Part model, mm, in its own coordinate system. Face numbers are marked on the shaded views. A direction names the side the tool comes from. Coordinates: 2 decimals unless noted, no trailing zeros. Loops run counter-clockwise (first coordinate to the right, second up) from the corner with the lowest first, then second, coordinate; pieces in that order, holes last. Notation, with made-up numbers: (72.25, 14.5) -> (120.25, 14.5) arc R7 ccw to (120.25, 26.5) -> close; hole circle Ø7 at (60, 3). An arc over 180 degrees is marked (long way). One line per item, written item: value. Start each with the question number.
from build123d import *

# Parameters (mm, degrees)
F0_W      = 1000
F0_H      = 2100
F1_DEPTH  = 800
F2_W      = 580
F2_H      = 1170
F3_DEPTH  = 350
F4_R      = 11
F5_DEPTH  = 40
F6_R      = 20
F7_DEPTH  = 5
F8_W      = 310
F8_H      = 200
F9_DEPTH  = 3
F10_W     = 100
F10_H     = 80
F11_DEPTH = 1
F12_W     = 880
F12_H     = 100
F13_DEPTH = 1150.001
F14_W     = 24
F14_H     = 100
F15_DEPTH = 25
F16_W     = 100
F16_H     = 50
F17_DEPTH = 2
F18_W     = 30
F18_H     = 175
F19_DEPTH = 4
F20_W     = 240
F20_H     = 130
F21_DEPTH = 1
F22_W     = 60
F22_H     = 25
F23_DEPTH = 0.1
F29_R     = 11
F30_DEPTH = 1


with BuildPart() as f1:
    # F0 (on Front) → F1 (new body)
    with BuildSketch(Plane.XZ):
        Rectangle(F0_W, F0_H)
    extrude(amount=-F1_DEPTH)

    # F2 (on face) → F3 (join)
    with BuildSketch(Plane(origin=(0, 800, 0), x_dir=(-1, 0, 0), z_dir=(0, 1, 0))):
        with Locations((0, 435)):
            Rectangle(F2_W, F2_H)
    extrude(amount=F3_DEPTH)

    # F4 (on face) → F5 (join)
    with BuildSketch(Plane.XZ):
        with Locations((0, 200)):
            Circle(F4_R)
    extrude(amount=F5_DEPTH)

    # F6 (on face) → F7 (join)
    with BuildSketch(Plane.XZ.offset(40)):
        with Locations((0, 200)):
            Circle(F6_R)
    extrude(amount=-F7_DEPTH)

    # F8 (on face) → F9 (join)
    with BuildSketch(Plane.XZ):
        with Locations((0, 410)):
            Rectangle(F8_W, F8_H)
    extrude(amount=F9_DEPTH)

    # F10 (on face) → F11 (cut)
    with BuildSketch(Plane.XZ):
        with Locations((-360, 50)):
            Rectangle(F10_W, F10_H)
    extrude(amount=-F11_DEPTH, mode=Mode.SUBTRACT)

    # F12 (on face) → F13 (cut, through all)
    with BuildSketch(Plane.XZ):
        with Locations((0, -1000)):
            Rectangle(F12_W, F12_H)
    extrude(amount=-F13_DEPTH, mode=Mode.SUBTRACT)

    # F14 (on face) → F15 (join)
    with BuildSketch(Plane.XZ):
        with Locations((480, 0)):
            Rectangle(F14_W, F14_H)
    extrude(amount=F15_DEPTH)

    # F16 (on face) → F17 (join)
    with BuildSketch(Plane.XZ):
        with Locations((-370, 945)):
            Rectangle(F16_W, F16_H)
    extrude(amount=F17_DEPTH)

    # F18 (on face) → F19 (join)
    with BuildSketch(Plane.XZ.offset(25)):
        with Locations((480, -29.5)):
            Rectangle(F18_W, F18_H)
    extrude(amount=F19_DEPTH)

    # F20 (on face) → F21 (join)
    with BuildSketch(Plane.XZ.offset(3)):
        with Locations((0, 408)):
            Rectangle(F20_W, F20_H)
    extrude(amount=F21_DEPTH)

    # F22 (on face) → F23 (cut)
    with BuildSketch(Plane.XZ.offset(4)):
        with Locations((-73, 444.5)):
            Rectangle(F22_W, F22_H)
        with Locations((10, 444.5)):
            Rectangle(F22_W, F22_H)
    extrude(amount=-F23_DEPTH, mode=Mode.SUBTRACT)

    # F26 (on plane+point) → F27 (revolve)
    with BuildSketch(Plane(origin=(0, 0, 393), x_dir=(1, 0, 0), z_dir=(0, 0, -1))):
        Polygon((-95.5, 4), (-73, 4), (-73, 26), (-83, 26), (-85, 16), (-95.5, 14), align=None)
    revolve(axis=Axis((-73, -17.4706345424, 393), (0, 1, 0)))

    # F26 (on plane+point) → F28 (revolve)
    with BuildSketch(Plane(origin=(0, 0, 393), x_dir=(1, 0, 0), z_dir=(0, 0, -1))):
        Polygon((-12.5, 4), (10, 4), (10, 26), (0, 26), (-2, 16), (-12.5, 14), align=None)
    revolve(axis=Axis((10, -12.9324262962, 393), (0, 1, 0)))

    # F29 (on face) → F30 (join)
    with BuildSketch(Plane.XZ.offset(4)):
        with Locations((83.5474357009, 438)):
            Circle(F29_R)
        with Locations((83.5474357009, 403)):
            Circle(F29_R)
    extrude(amount=F30_DEPTH)


solid = f1.part
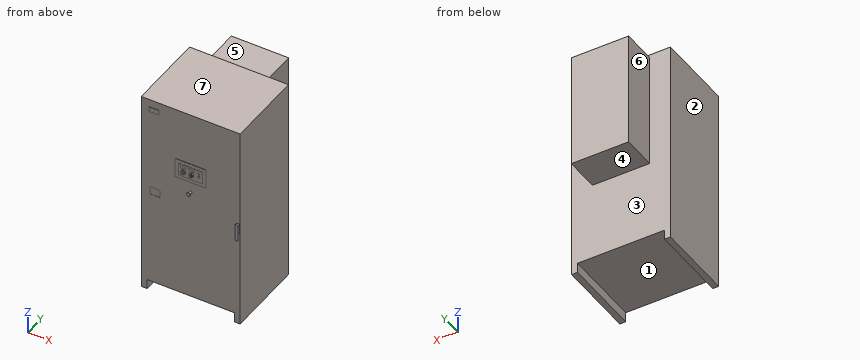
1) Probe line 1 (Y direction, x = -131.5, z = -407.5); line 2 (Z direction, x = 279, y = 645); line 3 (Y direction, x = 148.5, z = -118). List the from-to ranges inside material, lowest first. Write a range as from..to.
2) Slice it at D-D (x = 344). Give the cut face in (y, z).
3) Tool access for the marked faces 4, 5, 6 and 7: list every direction of +Z, -Z, +X, -X, +Y, -Y with a clear straight run to the whole face (end or side of a thin tool).
4) Pull direction X, two halves, no side cores. Call the marked faces 1, 2 and 3: +X half, -X half, draft (parallel to the pull), parting line (faces both ways), or undercut.
5) Pin check, flat tips, straight feed: pin 1 Ø3 at (x, y) = (-21.5, 805) entering from +Z; pin 2 Ø2.5 at (y, z) = (-1.5, 387.5) entering from +X; pin 3 Ø1.1 at (x, y) = (-3, -3.5) entering from -Z. Stop position of each tip, or through.
6) Slice it at C-C (z = -456.5). Give the cut face in (x, y), then the cut area to 3 significant figures.
7) Slice it at B-B (x = 191). Give the cut face in (y, z), then the cut area to 3 significant figures.
8) Slice it at A-A (z = 659). Give the cut face in (x, y).
Check sheet entries:
1. line 1: y = 0..800
1. line 2: z = -950..1050
1. line 3: y = 0..1150
2. outline: (0, -950) -> (800, -950) -> (800, 1050) -> (0, 1050) -> close
3. face 4: -Z, +X, -X, +Y
3. face 5: +Z, +X, -X, +Y
3. face 6: +Z, -Z, -X, +Y
3. face 7: +Z, +X, -X, +Y, -Y
4. face 1: undercut
4. face 2: -X half
4. face 3: draft
5. pin 1: stops at z = 1020
5. pin 2: stops at x = 155
5. pin 3: stops at z = 189.28
6. outline: (-500, 0) -> (500, 0) -> (500, 800) -> (-500, 800) -> close
6. area: 800,000 mm^2
7. outline: (0, -950) -> (800, -950) -> (800, -150) -> (1150, -150) -> (1150, 1020) -> (800, 1020) -> (800, 1050) -> (0, 1050) -> close
7. area: 2,010,000 mm^2
8. outline: (-500, 0) -> (500, 0) -> (500, 800) -> (290, 800) -> (290, 1150) -> (-290, 1150) -> (-290, 800) -> (-500, 800) -> close
